Verification items for the finished model (mm, model axes). Face numbers are marked on the shaded views. Coordinates: 2 decimals unless noted, no trailing zeros. Order: outer loops, then holes, each group sorted by start corner. A loop starts at its lowest first (then second) coordinate and runs counter-clockwise, first axis right, second up. Notation, with made-up numbers: (-17, 11.5) -> (38, 11.5) arc R27 cw to (38, 47.5) -> close; hole circle Ø1 at (7.25, 23). An arc over 180 degrees is marked (long way). Answer as CSV lines item,"result".
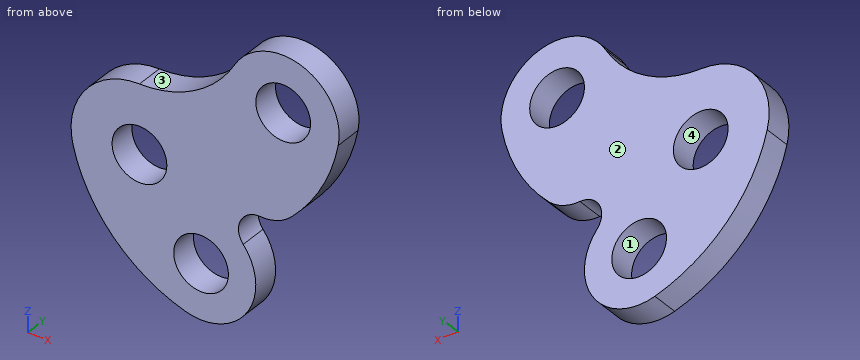
```python
from build123d import *

# Parameters (mm, degrees)
F0_R     = 10
F1_DEPTH = 10


with BuildPart() as f1:
    # F0 (on Front) → F1 (new body)
    with BuildSketch(Plane.XZ):
        with BuildLine():
            ThreePointArc((0, 25), (-19.664959, 15.436625), (-24.284847, -5.93685))
            ThreePointArc((-24.284847, -5.93685), (-9.512511, -33.001447), (16.750607, -49.155795))
            ThreePointArc((16.750607, -49.155795), (39.169931, -41.050494), (37.904534, -17.244596))
            ThreePointArc((37.904534, -17.244596), (36.990811, -9.071889), (44.120823, -4.974213))
            ThreePointArc((44.120823, -4.974213), (50.230306, -4.058588), (55.452633, -0.758367))
            ThreePointArc((55.452633, -0.758367), (66.51285, 13.90815), (72.617387, 31.233557))
            ThreePointArc((72.617387, 31.233557), (59.558682, 54.211204), (34.729726, 45.154442))
            ThreePointArc((34.729726, 45.154442), (20.077073, 30.403596), (0, 25))
        make_face()
        with Locations((22.5, -30)):
            Circle(F0_R, mode=Mode.SUBTRACT)
        Circle(F0_R, mode=Mode.SUBTRACT)
        with Locations((52.5, 35)):
            Circle(F0_R, mode=Mode.SUBTRACT)
    extrude(amount=F1_DEPTH)


solid = f1.part
```
Item 1: Section check B-B, the plane x = 22.5. Record the boundary of the cut face in (y, z).
Answer list:
outline,"(-10, -50) -> (0, -50) -> (0, -40) -> (-10, -40) -> close; (-10, -20) -> (0, -20) -> (0, 31.93) -> (-10, 31.93) -> close"
Item 2: Release check for a two-part mould opening along X. For the marked faces 1, 2, 3 and 4 record: +X half, -X half, draft (parallel to the pull), parting line (faces both ways), or undercut.
Answer list:
face 1,"undercut"
face 2,"draft"
face 3,"-X half"
face 4,"undercut"
Item 3: Section check A-A, the plane z = 27. Record the boundary of the cut face in (x, y).
Answer list:
outline,"(12.49, -10) -> (46.5, -10) -> (46.5, 0) -> (12.49, 0) -> close; (58.5, -10) -> (71.67, -10) -> (71.67, 0) -> (58.5, 0) -> close"
Item 4: Section check D-D, the plane z = 13.5. Record the boundary of the cut face in (x, y), plus the area to 3 significant figures.
Answer list:
outline,"(-21.04, -10) -> (66.29, -10) -> (66.29, 0) -> (-21.04, 0) -> close"
area,"873 mm2"
Item 5: Section check C-C, the plane y = -2. Record the boundary of the cut face in (x, z).
Answer list:
outline,"(-24.28, -5.94) arc R60 ccw to (16.75, -49.16) arc R20 ccw to (37.9, -17.24) arc R7.5 cw to (44.12, -4.97) arc R15 ccw to (55.45, -0.76) arc R60 ccw to (72.62, 31.23) arc R20.47 ccw to (34.73, 45.15) arc R40 cw to (0, 25) arc R25 ccw to start; hole circle Ø20 at (0, 0); hole circle Ø20 at (22.5, -30); hole circle Ø20 at (52.5, 35)"
Item 6: Depth check by flat-ended pin: pin 1 Ø18 at (x, z) = (52.5, 35) entering from -Y; pin 2 Ø6 at (x, y) = (34.5, -2.5) entering from -Z; pin 3 Ø1 at (x, y) = (56, -5.5) entering from -Z; pin 4 Ø6 at (x, y) = (36, -6.5) entering from +Z. Enter the tip coordinate at first touch or a pass-through.
Answer list:
pin 1,"through"
pin 2,"z = -47.86"
pin 3,"z = -0.71"
pin 4,"z = 50.38"
Item 7: Thickness scan on line 1 (Z direction, x = 38.5, y = -1.75); line 2 (X direction, y = -3.25, z = 32.5); line 3 (Z direction, x = 60.5, y = -8.25). Record the ranges inside material, lowest first.
Answer list:
line 1,"-42 to -18, -7.04 to 49.93"
line 2,"23.32 to 42.82, 62.18 to 72.81"
line 3,"4.8 to 29, 41 to 53.84"
